from build123d import *

# Parameters (mm, degrees)
SKETCH_1_R           = 21
EXTRUDE_1_DEPTH      = 39
SKETCH_2_R           = 13
EXTRUDE_2_DEPTH      = 2
SKETCH_4_R           = 5
EXTRUDE_3_DEPTH      = 25.3
CHAMFER_1_SIZE       = 0.5
SKETCH_8_R           = 1.5
CUT_EXTRUDE_7_DEPTH  = 10.3
MM_2_D               = 5
MM_2_DEPTH           = 10
MM_2_TIP             = 1.502151548
CUT_EXTRUDE_8_DEPTH  = 2
MM_1_D               = 4
MM_1_DEPTH           = 10
MM_1_TIP             = 1.201721238
SKETCH_23_W          = 4
SKETCH_23_H          = 0.5
CUT_EXTRUDE_12_DEPTH = 2
SKETCH_24_R          = 20
EXTRUDE_4_DEPTH      = 1
EXTRUDE_START        = 8
SKETCH_26_R          = 21
EXTRUDE_5_DEPTH      = 8
SKETCH_27_R          = 20
EXTRUDE_6_DEPTH      = 0.8
EXTRUDE_START_2      = 17.9
SKETCH_28_R          = 21
EXTRUDE_7_DEPTH      = 17.9
CHAMFER_2_SIZE       = 4
SKETCH_29_R          = 4
EXTRUDE_8_DEPTH      = 4.4
CUT_EXTRUDE_16_DEPTH = 2
CHAMFER_3_SIZE       = 0.2


with BuildPart() as part:
    # 草图1 → 凸台-拉伸1 (new body)
    with BuildSketch(Plane.XY):
        Circle(SKETCH_1_R)
    extrude(amount=EXTRUDE_1_DEPTH)

    # 草图2 → 凸台-拉伸2 (add)
    with BuildSketch(Plane.XY.offset(39)):
        Circle(SKETCH_2_R)
    extrude(amount=EXTRUDE_2_DEPTH)

    # 草图4 → 凸台-拉伸3 (add)
    with BuildSketch(Plane.XY.offset(41)):
        Circle(SKETCH_4_R)
    extrude(amount=EXTRUDE_3_DEPTH)

    # 倒角1
    chamfer_1_edges = [part.edges().sort_by_distance(p)[0] for p in [
        (-5, 0, 66.3),
    ]]
    chamfer(chamfer_1_edges, length=CHAMFER_1_SIZE)

    # 草图8 → 切除-拉伸7 (cut)
    with BuildSketch(Plane(origin=(0, -5, 0), x_dir=(1, 0, 0), z_dir=(0, 1, 0))):
        with Locations(Location((0, -56.3, 0), (0, 0, 90))):
            Circle(SKETCH_8_R)
    extrude(amount=CUT_EXTRUDE_7_DEPTH, mode=Mode.SUBTRACT)

    # 大小mm 暗销孔2
    with Locations(Plane.XY.offset(66.3)):
        with Locations((0, 0)):
            Hole(MM_2_D / 2, depth=MM_2_DEPTH)
            with Locations((0, 0, -(MM_2_DEPTH + MM_2_TIP / 2))):  # 118° drill point
                Cone(0, MM_2_D / 2, MM_2_TIP, mode=Mode.SUBTRACT)

    # 草图17 → 切除-拉伸8 (cut)
    with BuildSketch(Plane(origin=(0, 4, 0), x_dir=(1, 0, 0), z_dir=(0, 1, 0))):
        Polygon((0, -65.8), (-2, -65.8), (-2, -46.3), (0, -46.3), (2, -46.3), (2, -65.8), align=None)
    extrude(amount=CUT_EXTRUDE_8_DEPTH, mode=Mode.SUBTRACT)

    # 大小mm 暗销孔1
    with Locations(Plane(origin=(0, 17.5, 39), x_dir=(1, 0, 0), z_dir=(0, 0, 1))):
        with Locations((0, 0), (-17.5, -17.5), (17.5, -17.5), (0, -35)):
            Hole(MM_1_D / 2, depth=MM_1_DEPTH)
            with Locations((0, 0, -(MM_1_DEPTH + MM_1_TIP / 2))):  # 118° drill point
                Cone(0, MM_1_D / 2, MM_1_TIP, mode=Mode.SUBTRACT)

    # 草图23 → 切除-拉伸12 (cut)
    with BuildSketch(Plane(origin=(0, 4, 0), x_dir=(1, 0, 0), z_dir=(0, 1, 0))):
        with Locations((0, -66.05)):
            Rectangle(SKETCH_23_W, SKETCH_23_H)
    extrude(amount=CUT_EXTRUDE_12_DEPTH, mode=Mode.SUBTRACT)

    # 草图24 → 凸台-拉伸4 (add)
    with BuildSketch(Plane(origin=(0, 0, 0), x_dir=(-1, 0, 0), z_dir=(0, 0, -1))):
        with Locations(Location((0, 0, 0), (0, 0, 180))):
            Circle(SKETCH_24_R)
    extrude(amount=EXTRUDE_4_DEPTH)

    # 草图26 → 凸台-拉伸5 (add)
    with BuildSketch(Plane(origin=(0, 0, -1), x_dir=(-1, 0, 0), z_dir=(0, 0, -1)).offset(EXTRUDE_START)):
        with Locations(Location((0, 0, 0), (0, 0, 180))):
            Circle(SKETCH_26_R)
    extrude(amount=-EXTRUDE_5_DEPTH)

    # 草图27 → 凸台-拉伸6 (add)
    with BuildSketch(Plane(origin=(0, 0, -9), x_dir=(-1, 0, 0), z_dir=(0, 0, -1))):
        with Locations(Location((0, 0, 0), (0, 0, 180))):
            Circle(SKETCH_27_R)
    extrude(amount=EXTRUDE_6_DEPTH)

    # 草图28 → 凸台-拉伸7 (add)
    with BuildSketch(Plane(origin=(0, 0, -9.8), x_dir=(-1, 0, 0), z_dir=(0, 0, -1)).offset(EXTRUDE_START_2)):
        with Locations(Location((0, 0, 0), (0, 0, 180))):
            Circle(SKETCH_28_R)
    extrude(amount=-EXTRUDE_7_DEPTH)

    # 倒角2
    chamfer_2_edges = [part.edges().sort_by_distance(p)[0] for p in [
        (-21, 0, -27.7),
    ]]
    chamfer(chamfer_2_edges, length=CHAMFER_2_SIZE)

    # 草图29 → 凸台-拉伸8 (add)
    with BuildSketch(Plane(origin=(0, 0, -27.7), x_dir=(-1, 0, 0), z_dir=(0, 0, -1))):
        Circle(SKETCH_29_R)
    extrude(amount=EXTRUDE_8_DEPTH)

    # 草图30 → 切除-拉伸16 (cut)
    with BuildSketch(Plane(origin=(0, 4, 0), x_dir=(1, 0, 0), z_dir=(0, 1, 0))):
        Polygon((0, -46.3), (3, -46.3), (3, -66.3), (-3, -66.3), (-3, -46.3), align=None)
    extrude(amount=CUT_EXTRUDE_16_DEPTH, mode=Mode.SUBTRACT)

    # 倒角3
    chamfer_3_edges = [part.edges().sort_by_distance(p)[0] for p in [
        (2.5, 0, 66.3),
    ]]
    chamfer(chamfer_3_edges, length=CHAMFER_3_SIZE)


solid = part.part
For this review, take the finished solid that the model builds, in its own axes (mm). A direction names the side the tool comes from. Round coordinates to 2 decimals unless told otherwise and drop trailing zeros. Order: outer loops, then holes, each group sorted by start corner. A loop starts at its lowest first (then second) coordinate and runs counter-clockwise, first axis right, second up. Notation, with made-up numbers: M 72,29 L 127,29 A11 cw 127,41 Z; hole C -4.5,-9.5 d5. An arc over 180 degrees is marked long. Write each question's results on one line, items separated by ' | '. Start each with the question number.
1. To check wall thickness, follow L1, parallel to Y at x = 0, z = 32.5; L2, parallel to Y at x = 17.5, z = 32.5; L3, parallel to Z at x = -6.5, y = -15.5. State the ranges of each line that lie inside material, in increasing order. Write a range as [from, to].
2. Draft analysis for pull direction Z (two halves, no side actions). For faces 6 (the face through (20.03, 6.31, 19.23)), 7 (the face through (19, -8, 0)), 8 (the face through (-17.78, -0.21, 28.01)), state which applies: pulls with the +Z half, pulls with the -Z half, needs draft (parallel to the pull), parting line crosses it, or undercut.
3. Clearance check with flat-ended pins moving along their axes: pin 1 Ø12 at (y, z) = (9, -1.5) entering from +X; pin 2 Ø6.5 at (x, y) = (17.5, 0) entering from -Z; pin 3 Ø12.5 at (x, y) = (5.5, 8) entering from +Z; pin 4 Ø5 at (x, z) = (-1, 24.5) entering from +Y. State where each tip first meets the part, or that it passes through.
4. Tool access review of faces 1 (the face through (-15.9, -1.2, 33.9)), 2 (the face through (0.867, -3.905, -29.869)), 3 (the face through (20.03, -6.31, -16.85)), 4 (the face through (0, -3, 66.3)), 5 (the face through (-19.98, -0.88, -9.39)): name each direction out of +Z, -Z, +X, -X, +Y, -Y from which nothing blocks a thin tool from reaching the whole face with its end or side.
5. Add section A-A (z = 36). State the section outline as (x, y) points, then the cut area to 3 significant figures.
Output values:
1) L1: [-21, -19.5], [-15.5, 15.5], [19.5, 21] | L2: [-11.61, -2], [2, 11.61] | L3: [-27.7, 39]
2) face 6: needs draft | face 7: undercut | face 8: pulls with the +Z half
3) pin 1: x = 20.78 | pin 2: z = -27.7 | pin 3: z = 66.3 | pin 4: y = 21
4) face 1: +Z | face 2: -Z | face 3: +Z, -Z | face 4: +Z, +X, -X, +Y, -Y | face 5: none
5) outline: C 0,0 d42; hole C -17.5,0 d4; hole C 0,-17.5 d4; hole C 0,17.5 d4; hole C 17.5,0 d4 | area: 1,340 mm^2
